Autodesk Inventor part; units mm, degrees
ref_plane "YZ Plane" through (0, 0, 0) normal (1, 0, 0) x (0, 1, 0)
ref_plane "XZ Plane" through (0, 0, 0) normal (0, 1, 0) x (-1, 0, 0)
ref_plane "XY Plane" through (0, 0, 0) normal (0, 0, 1) x (1, 0, 0)
sketch "Sketch1" plane through (0, 0, 0) normal (0, 1, 0) x (-1, 0, 0)
  point P0 (0, 0)
sketch "Sketch2" plane through (0, 0, 0) normal (0, 1, 0) x (-1, 0, 0)
  line L0 (0.0816, -0.0238) -> (77.0816, -0.0238)
  line L1 (77.0816, -0.0238) -> (77.0816, -264.0238)
  line L2 (77.0816, -264.0238) -> (0.0816, -264.0238)
  line L3 (0.0816, -264.0238) -> (0.0816, -0.0238)
  line L4 (2.0816, -2.0238) -> (75.0816, -2.0238)
  line L5 (75.0816, -2.0238) -> (75.0816, -262.0238)
  line L6 (75.0816, -262.0238) -> (2.0816, -262.0238)
  line L7 (2.0816, -262.0238) -> (2.0816, -2.0238)
  line L8 (2.0816, -2.0238) -> (2.0816, -4.4588)
  line L9 (75.0816, -2.0238) -> (75.0816, -4.4588)
  line L10 (2.0816, -262.0238) -> (2.0816, -226.5538)
  circle A0 centre (72.3366, -4.2738) radius 2.25
  circle A1 centre (4.3316, -4.4588) radius 2.25
  circle A2 centre (4.3316, -226.5538) radius 2.25
  circle A3 centre (72.3366, -226.5538) radius 2.25
  dimension "d24" = 4.5
  dimension "d25" = 4.5
  dimension "d3" = 77
  dimension "d4" = 264
  dimension "d7" = 73
  dimension "d8" = 260
  dimension "d23" = 4.5
  dimension "d26" = 4.5
extrude "Extrusion1" add sketch "Sketch2" along normal blind 3 contours L0 L1 L2 L3 | A1 | A2 | A0 | L4 L5 L6 L7 | A3
sketch "Sketch3" plane through (-77.1633, 3, -264.0476) normal (0, 1, 0) x (1, 0, 0)
  line L0 (2.0816, -2.0238) -> (2.0816, -4.4588)
  line L1 (75.0816, -2.0238) -> (75.0816, -4.4588)
  circle A0 centre (72.3366, -4.2738) radius 2.25
  circle A1 centre (4.3316, -4.4588) radius 2.25
  circle A2 centre (4.3316, -226.5538) radius 2.25
  circle A3 centre (72.3366, -226.5538) radius 2.25
  dimension "d29" = 4.5
  dimension "d30" = 4.5
  dimension "d28" = 4.5
  dimension "d27" = 4.5
extrude "Extrusion3" add sketch "Sketch3" along normal blind 6
hole "Hole1" at (-4.8266, 9, -259.7738) direction (0, -1, 0) diameter 3 depth 4
hole "Hole2" at (-4.8266, 9, -37.4938) direction (0, -1, 0) diameter 3 depth 4
hole "Hole3" at (-72.8316, 9, -37.4938) direction (0, -1, 0) diameter 3 depth 4
hole "Hole4" at (-72.8316, 9, -259.5888) direction (0, -1, 0) diameter 3 depth 4
Source: CAD feature listing. Evaluate the final solid. Frame: model axes, mm. A direction names the side the tool comes from. Give positions to 0.01 mm unless a question says otherwise; leave off trailing zeros. Write each loop counter-clockwise with the first axis right and the second up, starting at its lowest first coordinate (ties: lowest second). Pieces come first, ordered by that corner, then holes.
1. Pull-direction query (Z, two-part tool) for faces 3 (the face through (-72, 9, -258)), 4 (the face through (-70.753, 5.958, -38.356)); classes: +Z half, -Z half, draft (parallel to the pull), parting line (faces both ways), or undercut.
2. Access query for faces 1 (the face through (-3.79, 5.96, -39.49)), 2 (the face through (-71, 9, -37)). Directions: +Z, -Z, +X, -X, +Y, -Y. A direction counts if a zero-diameter tool reaches every point of the face in a straight line with its end or side. Return the directions, or none.
3. First-contact query: pin 1 (1.8 mm diameter, centred on x = -4.83, z = -259.77, fed in from +Y); pin 2 (10 mm diameter, centred on x = -45, z = -237, fed in from +Y). Flat tips, straight axial feed; report the tip coordinate or a pass-through.
4. Section query B-B (z = -152.5). Return the cut outline in (x, y), then the cut area to 3 significant figures.
5. Section query C-C (x = -45). Return the cut outline in (y, z), then the cut area to 3 significant figures.
6. Section query A-A (y = 6.75). Return the cut outline in (x, z), then the cut area to 3 significant figures.
7. Material intervals for line 1 along Y through (x, z) = (-47, -86); line 2 along Z through (x, y) = (-72, 3.75), sorted ascending.
Output values:
1. face 3: draft
1. face 4: undercut
2. face 1: +Y
2. face 2: +Z, -Z, +X, -X, +Y
3. pin 1: stops at y = 5
3. pin 2: stops at y = 3
4. outline: (-77.08, 0) - (-0.08, 0) - (-0.08, 3) - (-77.08, 3) - close
4. area: 231 mm2
5. outline: (0, -264.02) - (3, -264.02) - (3, -0.02) - (0, -0.02) - close
5. area: 792 mm2
6. outline: circle Ø4.5 at (-72.83, -259.59); circle Ø4.5 at (-72.83, -37.49); circle Ø4.5 at (-4.83, -259.77); circle Ø4.5 at (-4.83, -37.49); hole circle Ø3 at (-72.83, -259.59); hole circle Ø3 at (-72.83, -37.49); hole circle Ø3 at (-4.83, -259.77); hole circle Ø3 at (-4.83, -37.49)
6. area: 35.3 mm2
7. line 1: y = 0 to 3
7. line 2: z = -261.68 to -257.5, -39.58 to -35.4
